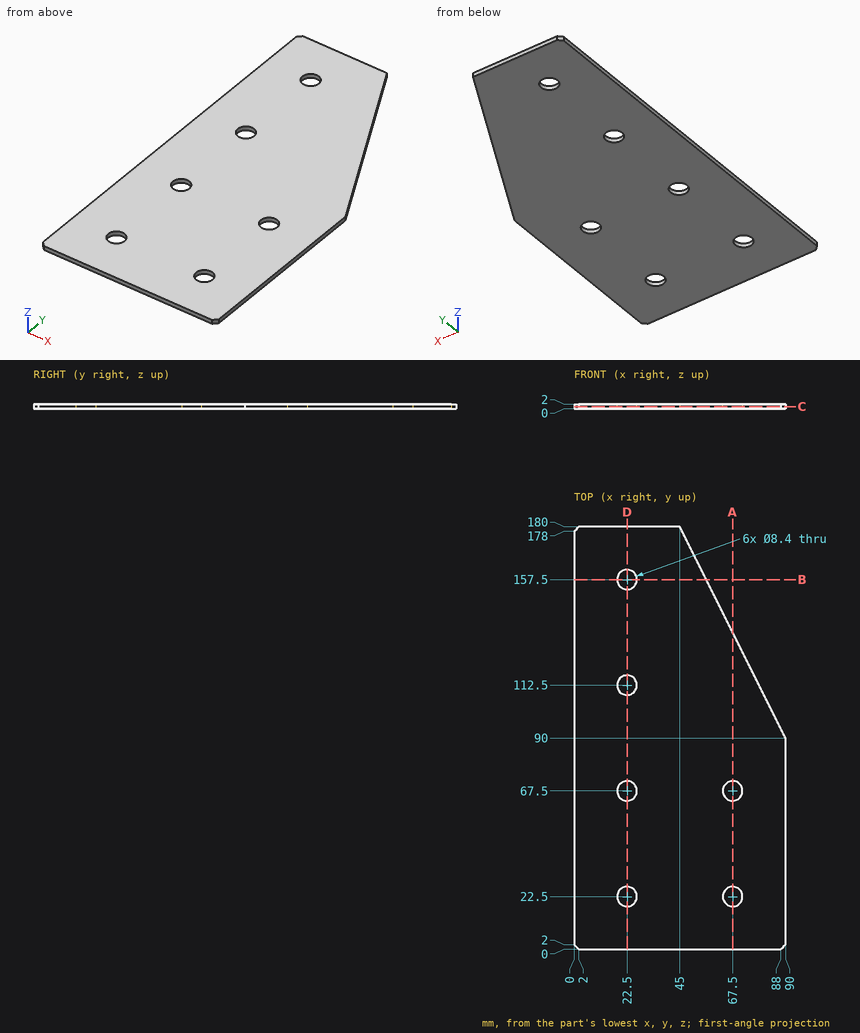
Source: three-view drawing plus pictorial views. Frame: mm from the lowest corner of the part. Give positions to 0.01 mm unless a question says otherwise; leave off trailing zeros. Write each loop counter-clockwise with the first axis right and the second up, starting at its lowest first coordinate (ties: lowest second). Pieces come first, ordered by that corner, then holes. Notation, with made-up numbers: (13.25, 20.5) - (69.25, 20.5) arc R14 cw to (69.25, 35.5) - close; hole circle Ø4 at (83.5, -39.5). An arc over 180 degrees is marked (long way). Write item = value, one per line. Start each with the question number.
Q1. Cut plane B-B, the plane y = 157.5. Return loops of the section in (x, z).
Q2. Material intervals for probe 1 along Y at (x, z) = (22.5, 1.3); probe 2 along X at (y, z) = (67.5, 1.5); probe 3 along Y at (x, z) = (67.5, 0.75), sorted ascending.
Q3. Cut plane D-D, the plane x = 22.5. Return loops of the section in (y, z).
Q4. Cut plane C-C, the plane z = 0.9. Return loops of the section in (x, y).
Q5. Cut plane A-A, the plane x = 67.5. Return loops of the section in (y, z).
Computed values:
q1.outline = (0, 0) - (18.3, 0) - (18.3, 2) - (0, 2) - close; (26.7, 0) - (56.25, 0) - (56.25, 2) - (26.7, 2) - close
q2.probe_1 = 0 to 18.3, 26.7 to 63.3, 71.7 to 108.3, 116.7 to 153.3, 161.7 to 180
q2.probe_2 = 0 to 18.3, 26.7 to 63.3, 71.7 to 90
q2.probe_3 = 0 to 18.3, 26.7 to 63.3, 71.7 to 135
q3.outline = (0, 0) - (18.3, 0) - (18.3, 2) - (0, 2) - close; (26.7, 0) - (63.3, 0) - (63.3, 2) - (26.7, 2) - close; (71.7, 0) - (108.3, 0) - (108.3, 2) - (71.7, 2) - close; (116.7, 0) - (153.3, 0) - (153.3, 2) - (116.7, 2) - close; (161.7, 0) - (180, 0) - (180, 2) - (161.7, 2) - close
q4.outline = (0, 2) - (2, 0) - (88, 0) - (90, 2) - (90, 90) - (45, 180) - (2, 180) - (0, 178) - close; hole circle Ø8.4 at (22.5, 22.5); hole circle Ø8.4 at (22.5, 67.5); hole circle Ø8.4 at (22.5, 112.5); hole circle Ø8.4 at (22.5, 157.5); hole circle Ø8.4 at (67.5, 22.5); hole circle Ø8.4 at (67.5, 67.5)
q5.outline = (0, 0) - (18.3, 0) - (18.3, 2) - (0, 2) - close; (26.7, 0) - (63.3, 0) - (63.3, 2) - (26.7, 2) - close; (71.7, 0) - (135, 0) - (135, 2) - (71.7, 2) - close
